Can you work these out from the drawing? Everything is in mm from the part's minimum corner. Give positions to 0.01 mm unless a question says otherwise; leave off trailing zeros. Write each loop counter-clockwise with the first axis right and the second up, starting at its lowest first coordinate (ties: lowest second). Pieces come first, ordered by that corner, then holes. Notation, with made-up numbers: (-15.5, 20.25) -> (31.5, 20.25) arc R13 ccw to (31.5, 35.25) -> close; hole circle Ø11 at (53.5, 16.5). An arc over 180 degrees is marked (long way). Return JSON: item names as keys, results as strings.
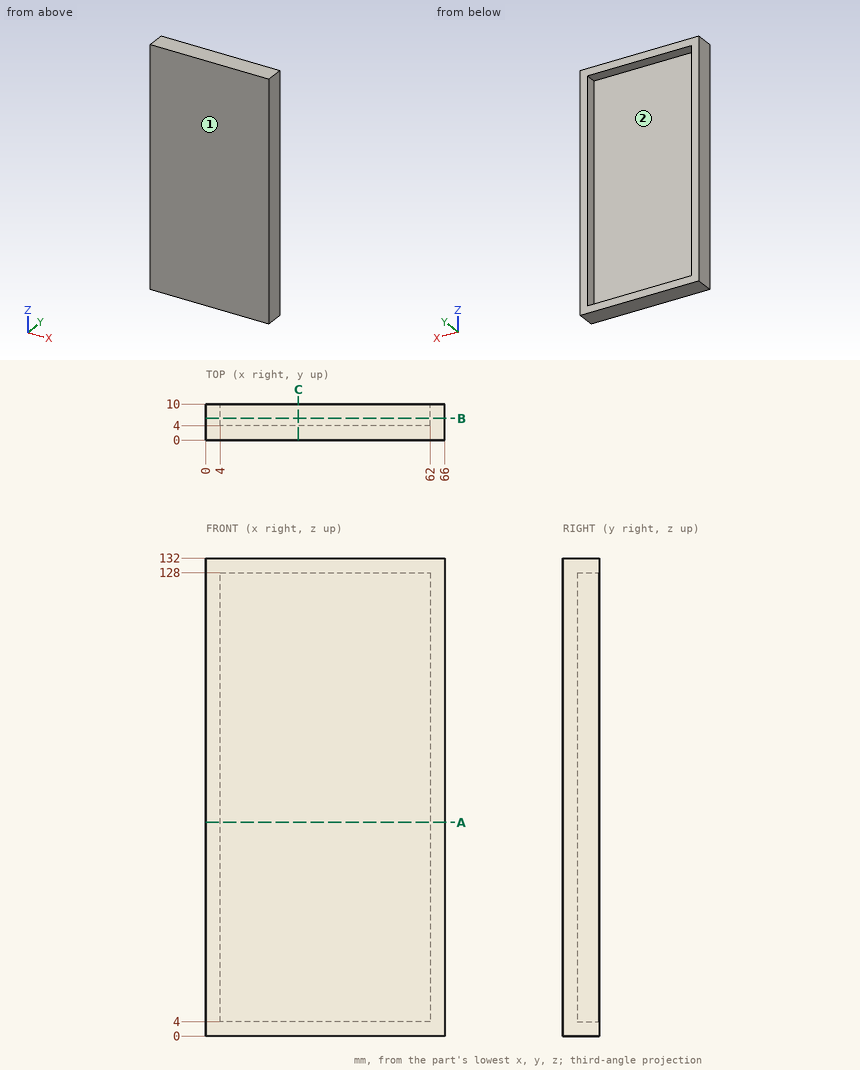
1. If I drill on line 1 (Z direction, x = 59, y = 8); line 2 (X direction, y = 5, z = 16.5); line 3 (Y direction, x = 40, z = 63.5), over which ranges is the centre line in solid material (lowest first)? Write a range as [from, to].
Taken from the geometry:
{"line 1": "z = [0, 4], [128, 132]", "line 2": "x = [0, 4], [62, 66]", "line 3": "y = [0, 4]"}
2. If we mould it in two halves opening along Z, with no side actions, what happens to the marked faces 1 and 2? For each: released by +Z, released by -Z, zero draft, split by the parting line, or undercut.
Taken from the geometry:
{"face 1": "zero draft", "face 2": "undercut"}
3. Suppose I cut it at A-A, the plane z = 59. List the corners of the cut face in (x, y) for me, and give its area (3 significant figures).
Taken from the geometry:
{"outline": "(0, 0) -> (66, 0) -> (66, 10) -> (62, 10) -> (62, 4) -> (4, 4) -> (4, 10) -> (0, 10) -> close", "area": "312 mm²"}
4. Suppose I cut it at B-B, the plane y = 6. List the corners of the cut face in (x, z) for me, and give its area (3 significant figures).
Taken from the geometry:
{"outline": "(0, 0) -> (66, 0) -> (66, 132) -> (0, 132) -> close; hole (4, 4) -> (62, 4) -> (62, 128) -> (4, 128) -> close", "area": "1,520 mm²"}
5. For pin 1 Ø1 at (x, z) = (45.5, 32.5) entering from +Y, with a flat end and sliding along its axis, tell me the tip position at first contact or that it passes through.
Taken from the geometry:
{"pin 1": "stops at y = 4"}
6. Suppose I cut it at C-C, the plane x = 25.5. List the corners of the cut face in (y, z) for me.
Taken from the geometry:
{"outline": "(0, 0) -> (10, 0) -> (10, 4) -> (4, 4) -> (4, 128) -> (10, 128) -> (10, 132) -> (0, 132) -> close"}
